Part model, mm, in its own coordinate system. Round coordinates to 2 decimals unless told otherwise and drop trailing zeros. Order: outer loops, then holes, each group sorted by start corner. A loop starts at its lowest first (then second) coordinate and runs counter-clockwise, first axis right, second up. Notation, with made-up numbers: (72, 66.5) - (98, 66.5) arc R20 ccw to (98, 102.5) - close; hole circle Ø2 at (54, 78). An arc over 180 degrees is marked (long way). Return JSON: item names as keys, results as strings. Group by question number.
Item 1: Saw through at B-B on y = 34.5. List the corners of the cut face in (x, z).
Item 2: Probe probe 1 along X at (y, z) = (0, 3.5); probe 2 along Y at (x, z) = (31.5, 3.75); probe 3 along X at (y, z) = (55.5, 2.5). List the from-to ranges inside material, lowest first.
Item 3: Saw through at C-C on y = -60. List the corners of the cut face in (x, z), and give its area (3 significant figures).
Item 4: Drop flat-ended pins along their axis: pin 1 (3.5 mm diameter, centred on x = 32.04, y = -55.5, fed in from +Z); pin 2 (2 mm diameter, centred on y = -56, z = 5, fed in from -X) (3 decimals); pin 3 (2 mm diameter, centred on x = -32.04, y = 55.5, fed in from -Z). Give the stop position or say it passes through.
Item 5: Saw through at A-A on z = 4.5. List the corners of the cut face in (x, y).
Autodesk Fusion 360 part; units mm, degrees
sketch "Sketch1" plane through (0, 0, 0) normal (0, 0, 1) x (1, 0, 0)
  line L0 (44.7446, 77.5) -> (-44.7446, 77.5)
  line L1 (-44.7446, 77.5) -> (-89.4893, 0)
  line L2 (-89.4893, 0) -> (-44.7446, -77.5)
  line L3 (-44.7446, -77.5) -> (44.7446, -77.5)
  line L4 (44.7446, -77.5) -> (89.4893, 0)
  line L5 (89.4893, 0) -> (44.7446, 77.5)
  dimension "d1" = 77.5
extrude "Extrude1" add sketch "Sketch1" along normal blind 7
sketch "Sketch2" plane through (0, 0, 7) normal (0, 0, 1) x (-1, 0, 0)
  line L0 (-89.4893, 0) -> (-44.7446, -77.5)
  line L1 (-44.7446, -77.5) -> (44.7446, -77.5)
  line L2 (44.7446, -77.5) -> (89.4893, 0)
  line L3 (89.4893, 0) -> (44.7446, 77.5)
  line L4 (44.7446, 77.5) -> (-44.7446, 77.5)
  line L5 (-44.7446, 77.5) -> (-89.4893, 0)
  line L6 (-32.0429, -77.5) -> (-32.0429, -55.5) construction
  line L7 (-51.0955, -66.5) -> (-32.0429, -55.5) construction
  line L8 (51.0955, -66.5) -> (32.0429, -55.5) construction
  line L9 (32.0429, -77.5) -> (32.0429, -55.5) construction
  line L10 (-83.1384, -11) -> (-64.0859, 0) construction
  line L11 (-83.1384, 11) -> (-64.0859, 0) construction
  line L12 (-32.0429, -77.5) -> (-32.0429, -55.5) construction
  line L13 (-51.0955, -66.5) -> (-32.0429, -55.5) construction
  line L14 (83.1384, 11) -> (64.0859, 0) construction
  line L15 (83.1384, -11) -> (64.0859, 0) construction
  line L16 (32.0429, 77.5) -> (32.0429, 55.5) construction
  line L17 (51.0955, 66.5) -> (32.0429, 55.5) construction
  line L18 (83.1384, 11) -> (64.0859, 0) construction
  line L19 (83.1384, -11) -> (64.0859, 0) construction
  line L20 (-51.0955, 66.5) -> (-32.0429, 55.5) construction
  line L21 (-32.0429, 77.5) -> (-32.0429, 55.5) construction
  circle A0 centre (-32.0429, 55.5) radius 1.5
  circle A1 centre (-64.0859, 0) radius 1.5
  circle A2 centre (-32.0429, -55.5) radius 1.5
  circle A3 centre (32.0429, -55.5) radius 1.5
  circle A4 centre (64.0859, 0) radius 1.5
  circle A5 centre (32.0429, 55.5) radius 1.5
  dimension "d4" = 22
  dimension "d5" = 22
  dimension "d6" = 22
  dimension "d7" = 22
  dimension "d8" = 22
  dimension "d9" = 22
  dimension "d10" = 22
  dimension "d11" = 22
  dimension "d12" = 22
  dimension "d13" = 22
  dimension "d14" = 22
  dimension "d15" = 22
  dimension "d16" = 22
  dimension "d17" = 22
  dimension "d18" = 22
  dimension "d19" = 22
  dimension "d20" = 3
  dimension "d21" = 3
  dimension "d22" = 3
  dimension "d23" = 3
  dimension "d24" = 3
  dimension "d25" = 3
hole "Hole1" at (32.0429, 55.5, 7) at (64.0859, 0, 7) at (32.0429, -55.5, 7) at (-32.0429, -55.5, 7) at (-32.0429, 55.5, 7) at (-64.0859, 0, 7) direction (0, 0, -1) diameter 2.529 end through all
Filled in:
{
 "1": {"outline": "(-69.57, 0) - (69.57, 0) - (69.57, 7) - (-69.57, 7) - close"},
 "2": {"probe 1": "x = -89.49 to -65.35, -62.82 to 62.82, 65.35 to 89.49", "probe 2": "y = -77.5 to -56.64, -54.36 to 54.36, 56.64 to 77.5", "probe 3": "x = -57.45 to -33.31, -30.78 to 30.78, 33.31 to 57.45"},
 "3": {"outline": "(-54.85, 0) - (54.85, 0) - (54.85, 7) - (-54.85, 7) - close", "area": "768 mm^2"},
 "4": {"pin 1": "stops at z = 7", "pin 2": "stops at x = -57.735", "pin 3": "passes through"},
 "5": {"outline": "(-89.49, 0) - (-44.74, -77.5) - (44.74, -77.5) - (89.49, 0) - (44.74, 77.5) - (-44.74, 77.5) - close; hole circle Ø2.53 at (-64.09, 0); hole circle Ø2.53 at (-32.04, -55.5); hole circle Ø2.53 at (-32.04, 55.5); hole circle Ø2.53 at (32.04, -55.5); hole circle Ø2.53 at (32.04, 55.5); hole circle Ø2.53 at (64.09, 0)"}
}
